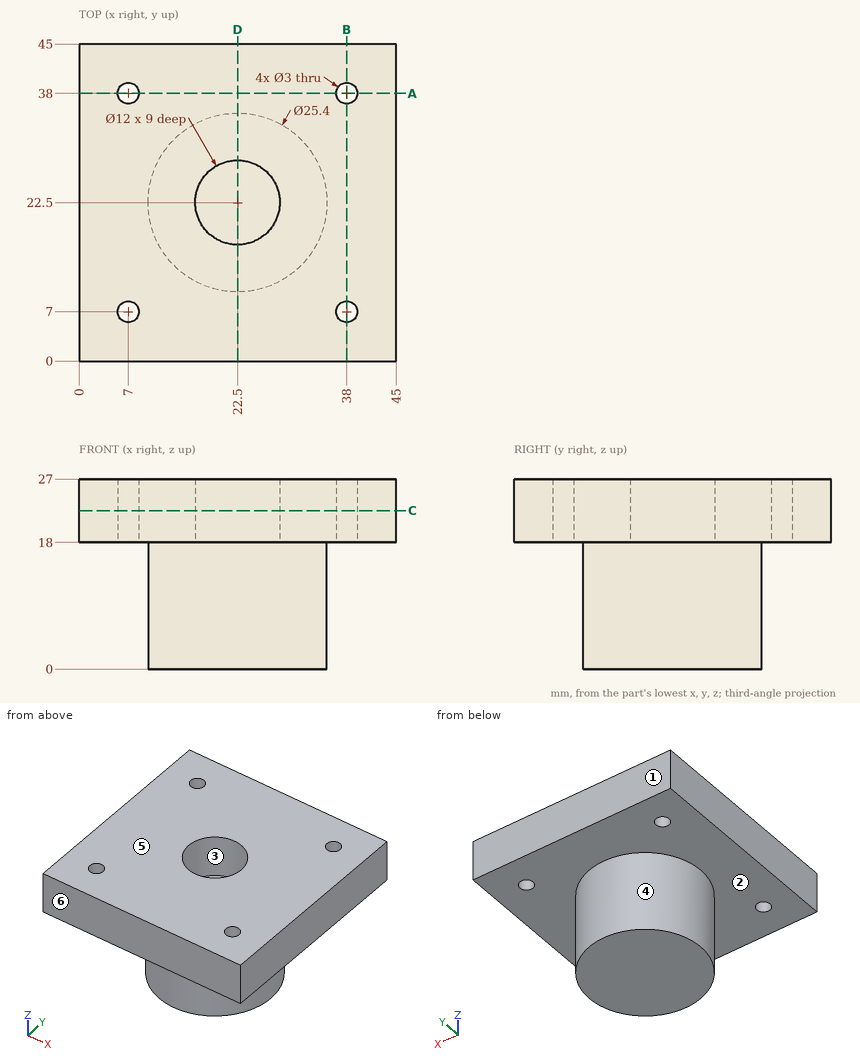
The drawing under review shows one solid part. Ordinate dimensions are in mm from its lowest x, y, z. A direction names the side the tool comes from. Coordinates: 2 decimals unless noted, no trailing zeros. Write each loop counter-clockwise with the first axis right and the second up, starting at its lowest first coordinate (ties: lowest second). Pieces come first, ordered by that corner, then holes. Notation, with made-up numbers: M -2.5,42 L 31.5,42 A23 cw 31.5,68 Z; hole C -20,41.5 d2. An arc over 180 degrees is marked long. Answer as a JSON object with one key per item and string values.
Item 1: Wall thickness on probe 1 along X at (y, z) = (7, 24.75); probe 2 along X at (y, z) = (22.5, 22.5): over which ranges is each line inside the solid? List them lowest first.
Outcome:
{"probe 1": "0 to 5.5, 8.5 to 36.5, 39.5 to 45", "probe 2": "0 to 16.5, 28.5 to 45"}
Item 2: Add section C-C, the plane z = 22.5. Give the boundary of the cut face in (x, y).
Outcome:
{"outline": "M 0,0 L 45,0 L 45,45 L 0,45 Z; hole C 7,7 d3; hole C 7,38 d3; hole C 22.5,22.5 d12; hole C 38,7 d3; hole C 38,38 d3"}
Item 3: Add section A-A, the plane y = 38. Give the boundary of the cut face in (x, z), and give its area (3 significant figures).
Outcome:
{"outline": "M 0,18 L 5.5,18 L 5.5,27 L 0,27 Z; M 8.5,18 L 36.5,18 L 36.5,27 L 8.5,27 Z; M 39.5,18 L 45,18 L 45,27 L 39.5,27 Z", "area": "351 mm²"}
Item 4: Draft analysis for pull direction Y (two halves, no side actions). For the marked faces 3, 4, 5 and 6, state which applies: pulls with the +Y half, pulls with the -Y half, needs draft (parallel to the pull), parting line crosses it, or undercut.
Outcome:
{"face 3": "undercut", "face 4": "parting line crosses it", "face 5": "needs draft", "face 6": "pulls with the -Y half"}
Item 5: Add section D-D, the plane x = 22.5. Give the boundary of the cut face in (y, z), and give its area (3 significant figures).
Outcome:
{"outline": "M 0,18 L 9.8,18 L 9.8,0 L 35.2,0 L 35.2,18 L 45,18 L 45,27 L 28.5,27 L 28.5,18 L 16.5,18 L 16.5,27 L 0,27 Z", "area": "754 mm²"}
Item 6: Insertion check: pin 1 Ø3 at (y, z) = (39.5, 15.5) entering from +X; pin 2 Ø6 at (x, y) = (24.5, 21) entering from +Z; pin 3 Ø8 at (y, z) = (36, 11.5) entering from +X; pin 4 Ø12 at (y, z) = (29, 5) entering from -X. Each pin has a flat end and moves straight along its axis. Give the tip position at first contact, or say it passes through.
Outcome:
{"pin 1": "through", "pin 2": "z = 18", "pin 3": "x = 30.93", "pin 4": "x = 9.81"}
Item 7: Machinability: for the marked faces 1 and 2, which of the approach directions +Z, -Z, +X, -X, +Y, -Y give a long, thin tool a straight path to every point of the face, cutting with its end or side? Answer none if there is none.
Outcome:
{"face 1": "+Z, -Z, +X, -X, +Y", "face 2": "-Z"}
